Autodesk Fusion 360 part; units mm, degrees
sketch "Box" plane through (0, 0, 0) normal (0, 0, 1) x (1, 0, 0)
  line L0 (55, 25) -> (-55, 25)
  line L1 (-55, 25) -> (-55, -25)
  line L2 (-55, -25) -> (55, -25)
  line L3 (55, -25) -> (55, 25)
  line L4 (55, 25) -> (-55, -25) construction
  line L5 (-55, 25) -> (55, -25) construction
  line L6 (56, -26) -> (-56, -26)
  line L7 (-56, -26) -> (-56, 26)
  line L8 (-56, 26) -> (56, 26)
  line L9 (56, 26) -> (56, -26)
  line L10 (56, -26) -> (-56, 26) construction
  line L11 (-56, -26) -> (56, 26) construction
  dimension "d2" = 110
  dimension "d3" = 50
  dimension "d4" = 112
  dimension "d5" = 52
extrude "Extrude1" add sketch "Box" along normal blind 55
fillet "Fillet1" radius 1 4 edges at (56, -26, 27.5) (-56, -26, 27.5) (56, 26, 27.5) (-56, 26, 27.5)
fillet "Fillet2" radius 1 4 edges at (55, -25, 27.5) (55, 25, 27.5) (-55, 25, 27.5) (-55, -25, 27.5)
ref_plane "WorkPlane1" through (0, 0, 55) normal (0, 0, 1) x (1, 0, 0)
sketch "Lid" plane through (0, 0, 55) normal (0, 0, 1) x (1, 0, 0)
  line L0 (55, -26) -> (-55, -26)
  line L1 (-56, -25) -> (-56, 25)
  line L2 (-55, 26) -> (55, 26)
  line L3 (56, 25) -> (56, -25)
  line L4 (56, -26) -> (-56, 26) construction
  line L5 (-56, -26) -> (56, 26) construction
  arc A0 (-55, 26) -> (-56, 25) centre (-55, 25) ccw
  arc A1 (56, 25) -> (55, 26) centre (55, 25) ccw
  arc A2 (55, -26) -> (56, -25) centre (55, -25) ccw
  arc A3 (-56, -25) -> (-55, -26) centre (-55, -25) ccw
  dimension "d13" = 112
  dimension "d14" = 52
  dimension "d15" = 1
  dimension "d16" = 1
  dimension "d17" = 1
  dimension "d18" = 1
extrude "Extrude2" add sketch "Lid" along normal blind 2
fillet "Fillet3" radius 1 8 edges at (0, 26, 57) (-55.7071, 25.7071, 57) (-56, 0, 57) (-55.7071, -25.7071, 57) (0, -26, 57) (55.7071, -25.7071, 57) (56, 0, 57) (55.7071, 25.7071, 57)
sketch "230 plug" plane through (0, 0, 57) normal (0, 0, 1) x (-1, 0, 0)
  line L0 (-55, -25) -> (55, -25)
  line L1 (55, -25) -> (55, 25)
  line L2 (55, 25) -> (-55, 25)
  line L3 (-55, 25) -> (-55, -25)
  line L4 (8.143, -13.9073) -> (-33.857, -13.9073)
  line L5 (-33.857, 14.0927) -> (8.143, 14.0927)
  line L6 (8.143, 14.0927) -> (8.143, -13.9073)
  line L7 (8.143, -13.9073) -> (-33.857, 14.0927) construction
  line L8 (-33.857, -13.9073) -> (8.143, 14.0927) construction
  line L9 (-33.857, 14.0927) -> (-40.2209, 7.7287)
  line L10 (-33.857, 14.0927) -> (-12.0333, 14.0927) construction
  line L11 (-33.857, -13.9073) -> (-40.2209, -7.5434)
  line L12 (-33.857, -13.9073) -> (-12.0333, -13.9073) construction
  line L13 (-40.2209, -7.5434) -> (-40.2209, 7.7287)
  point P0 (-12.857, 0.0927)
  dimension "d32" = 28
  dimension "d33" = 42
  dimension "d34" = 135
  dimension "d35" = 9
  dimension "d36" = 135
  dimension "d37" = 9
extrude "Extrude3" cut sketch "230 plug" against normal blind 2 contours L4 L5 L6 L9 L11 L13
ref_plane "WorkPlane2" through (0, 0, 55) normal (0, 0, -1) x (-1, 0, 0)
sketch "Screw Holes" plane through (0, 0, 55) normal (0, 0, -1) x (1, 0, 0)
  line L0 (-8.143, 14.0927) -> (-8.143, -13.9073)
  circle A0 centre (13.857, -19.9073) radius 1.5
  line L1 (-8.143, -13.9073) -> (13.857, -13.9073)
  line L2 (13.857, -13.9073) -> (13.857, -19.9073)
  circle A1 centre (13.857, -19.9073) radius 3.5
  line L3 (-8.143, 14.0927) -> (13.857, 14.0927)
  line L4 (13.857, 14.0927) -> (13.857, 20.0927)
  circle A2 centre (13.857, 20.0927) radius 3.5
  circle A3 centre (13.857, 20.0927) radius 1.5
  dimension "d44" = 3
  dimension "d45" = 22
  dimension "d46" = 6
  dimension "d47" = 7
  dimension "d49" = 22
  dimension "d50" = 6
  dimension "d51" = 7
  dimension "d52" = 3
extrude "Extrude5" add sketch "Screw Holes" along normal blind 20
extrude "Extrude6" cut sketch "Screw Holes" against normal blind 2 contours A0 | A3
sketch "XT60 plug 1" plane through (0, 0, 55) normal (0, 0, -1) x (1, 0, 0)
  circle A0 centre (13.857, -19.9073) radius 3.5
  line L0 (40.2209, 7.7287) -> (40.2209, -7.5434)
  line L1 (40.2209, -7.5434) -> (33.857, -13.9073)
  line L2 (33.857, -13.9073) -> (-8.143, -13.9073)
  line L3 (-8.143, -13.9073) -> (-8.143, 14.0927)
  line L4 (-8.143, 14.0927) -> (33.857, 14.0927)
  line L5 (33.857, 14.0927) -> (40.2209, 7.7287)
  arc A1 (-54, 25) -> (-55, 24) centre (-54, 24) ccw
  line L6 (-55, 24) -> (-55, -24)
  arc A2 (-55, -24) -> (-54, -25) centre (-54, -24) ccw
  line L7 (-54, -25) -> (54, -25)
  arc A3 (54, -25) -> (55, -24) centre (54, -24) ccw
  line L8 (55, -24) -> (55, 24)
  arc A4 (55, 24) -> (54, 25) centre (54, 24) ccw
  line L9 (54, 25) -> (-54, 25)
  circle A5 centre (13.857, 20.0927) radius 3.5
  line L10 (-50.4445, 8.0625) -> (-42.2445, 8.0625)
  line L11 (-42.2445, -5.4375) -> (-44.8962, -8.0891)
  line L12 (-50.4445, -5.4375) -> (-47.7929, -8.0891)
  line L13 (-47.7929, -8.0891) -> (-44.8962, -8.0891)
  line L14 (-37.9445, 8.0625) -> (-29.7445, 8.0625)
  line L15 (-29.7445, 8.0625) -> (-29.7445, -5.4375)
  line L16 (-29.7445, -5.4375) -> (-32.3962, -8.0891)
  line L17 (-37.9445, -5.4375) -> (-35.2929, -8.0891)
  line L18 (-35.2929, -8.0891) -> (-32.3962, -8.0891)
  line L19 (-17.2445, 8.0625) -> (-25.4445, 8.0625)
  line L20 (-25.4445, 8.0625) -> (-25.4445, -5.4375)
  line L21 (-25.4445, -5.4375) -> (-22.7929, -8.0891)
  line L22 (-17.2445, -5.4375) -> (-19.8962, -8.0891)
  line L23 (-22.7929, -8.0891) -> (-19.8962, -8.0891)
  line L24 (-42.2445, -5.4375) -> (-42.2445, 8.0625)
  line L25 (-37.9445, -5.4375) -> (-37.9445, 8.0625)
  line L26 (-17.2445, -5.4375) -> (-17.2445, 8.0625)
  line L27 (-50.4445, 8.0625) -> (-50.4445, -5.4375)
  line L28 (-42.2445, 1.3125) -> (-37.9445, 1.3125)
  line L29 (-29.7445, 1.3125) -> (-25.4445, 1.3125)
  dimension "d70" = 3.75
  dimension "d71" = 3.75
  dimension "d72" = 8.2
  dimension "d75" = 3.75
  dimension "d76" = 3.75
  dimension "d79" = 8.2
  dimension "d80" = 13.5
  dimension "d81" = 3.75
  dimension "d83" = 3.75
  dimension "d89" = 8.2
  dimension "d91" = 4.3
extrude "Extrude7" cut sketch "XT60 plug 1" against normal blind 2 contours L19 L20 L21 L22 L23 L26 | L14 L15 L16 L17 L18 L25 | L10 L11 L12 L13 L24 L27
sketch "Sketch7" plane through (0, 0, 55) normal (0, 0, -1) x (1, 0, 0)
  line L0 (-47.7929, -8.0891) -> (-50.4445, -5.4375)
  line L1 (-50.4445, 8.0625) -> (-42.2445, 8.0625)
  line L2 (-42.2445, 8.0625) -> (-42.2445, -5.4375)
  line L3 (-42.2445, -5.4375) -> (-44.8962, -8.0891)
  line L4 (-44.8962, -8.0891) -> (-47.7929, -8.0891)
  line L5 (-29.7445, -5.4375) -> (-32.3962, -8.0891)
  line L6 (-32.3962, -8.0891) -> (-35.2929, -8.0891)
  line L7 (-35.2929, -8.0891) -> (-37.9445, -5.4375)
  line L8 (-37.9445, -5.4375) -> (-37.9445, 8.0625)
  line L9 (-37.9445, 8.0625) -> (-29.7445, 8.0625)
  line L10 (-29.7445, 8.0625) -> (-29.7445, -5.4375)
  line L11 (-25.4445, 8.0625) -> (-17.2445, 8.0625)
  line L12 (-17.2445, 8.0625) -> (-17.2445, -5.4375)
  line L13 (-17.2445, -5.4375) -> (-19.8962, -8.0891)
  line L14 (-19.8962, -8.0891) -> (-22.7929, -8.0891)
  line L15 (-22.7929, -8.0891) -> (-25.4445, -5.4375)
  line L16 (-25.4445, -5.4375) -> (-25.4445, 8.0625)
  circle A0 centre (13.857, -19.9073) radius 3.5
  line L17 (40.2209, 7.7287) -> (40.2209, -7.5434)
  line L18 (40.2209, -7.5434) -> (33.857, -13.9073)
  line L19 (33.857, -13.9073) -> (-8.143, -13.9073)
  line L20 (-8.143, -13.9073) -> (-8.143, 14.0927)
  line L21 (-8.143, 14.0927) -> (33.857, 14.0927)
  line L22 (33.857, 14.0927) -> (40.2209, 7.7287)
  arc A1 (-54, 25) -> (-55, 24) centre (-54, 24) ccw
  line L23 (-55, 24) -> (-55, -24)
  arc A2 (-55, -24) -> (-54, -25) centre (-54, -24) ccw
  line L24 (-54, -25) -> (54, -25)
  arc A3 (54, -25) -> (55, -24) centre (54, -24) ccw
  line L25 (55, -24) -> (55, 24)
  arc A4 (55, 24) -> (54, 25) centre (54, 24) ccw
  line L26 (54, 25) -> (-54, 25)
  circle A5 centre (13.857, 20.0927) radius 3.5
  line L27 (-15.2847, -9.9279) -> (-52.5832, -9.9279)
  line L28 (-52.5832, -9.9279) -> (-52.5832, 10.117)
  line L29 (-52.5832, 10.117) -> (-15.2847, 10.117)
  line L30 (-15.2847, 10.117) -> (-15.2847, -9.9279)
  line L31 (-15.2847, -9.9279) -> (-52.5832, 10.117) construction
  line L32 (-52.5832, -9.9279) -> (-15.2847, 10.117) construction
  line L33 (-50.4445, -5.4375) -> (-50.4445, 8.0625)
  point P0 (-33.934, 0.0945)
extrude "Extrude8" add sketch "Sketch7" along normal blind 14 contours L27 L28 L29 L30
extrude "Extrude4" [suppressed]
Build history of the part. All positions in model axes, mm. A direction names the side the tool comes from. Round coordinates to 2 decimals unless told otherwise and drop trailing zeros. Write each loop counter-clockwise with the first axis right and the second up, starting at its lowest first coordinate (ties: lowest second). Pieces come first, ordered by that corner, then holes. Notation, with made-up numbers: (-20, 25.25) -> (20, 25.25) arc R8 cw to (20, 30.25) -> close; hole circle Ø4 at (-35.5, 27). An arc over 180 degrees is marked (long way). Write item = value, one per line.
(1) Band-saw the part on C-C (z = 16.5). Give the cut face in (x, y), then the cut area to 3 significant figures.
Answer:
outline = (-56, -25) arc R1 ccw to (-55, -26) -> (55, -26) arc R1 ccw to (56, -25) -> (56, 25) arc R1 ccw to (55, 26) -> (-55, 26) arc R1 ccw to (-56, 25) -> close; hole (-55, -24) arc R1 ccw to (-54, -25) -> (54, -25) arc R1 ccw to (55, -24) -> (55, 24) arc R1 ccw to (54, 25) -> (-54, 25) arc R1 ccw to (-55, 24) -> close
area = 324 mm2
(2) Tool access for faces 3 (the face through (-0.3, 25.2, 0)), 4 (the face through (-46, -8.062, 49)), 5 (the face through (-34, -10.117, 48)): list every direction of +Z, -Z, +X, -X, +Y, -Y with a clear straight run to the whole face (end or side of a thin tool).
Answer:
face_3 = -Z, +X, -X, +Y, -Y
face_4 = +Z, -Z
face_5 = -Z
(3) Two-plate mould, pull along Y, no slides. Class faces 1 (the face through (56, 0, 28)), 2 (the face through (-34, 9.928, 48)): pulls with the +Y half, pulls with the -Y half, needs draft (parallel to the pull), parting line crosses it, or undercut.
Answer:
face_1 = needs draft
face_2 = undercut
(4) Flat gauge pins, fed straight in: pin 1 (3.5 mm diameter, centred on x = 14.5, y = -21.5, fed in from -Z); pin 2 (6 mm diameter, centred on x = -40, y = 2, fed in from -Z). Where does each tip first touch, or does it go through?
Answer:
pin_1 = 35
pin_2 = 41
(5) Band-saw the part on D-D (z = 38.5). Give the cut face in (x, y), then the cut area to 3 significant figures.
Answer:
outline = (-56, -25) arc R1 ccw to (-55, -26) -> (55, -26) arc R1 ccw to (56, -25) -> (56, 25) arc R1 ccw to (55, 26) -> (-55, 26) arc R1 ccw to (-56, 25) -> close; circle Ø7 at (13.86, -20.09); circle Ø7 at (13.86, 19.91); hole (-55, -24) arc R1 ccw to (-54, -25) -> (54, -25) arc R1 ccw to (55, -24) -> (55, 24) arc R1 ccw to (54, 25) -> (-54, 25) arc R1 ccw to (-55, 24) -> close; hole circle Ø3 at (13.86, -20.09); hole circle Ø3 at (13.86, 19.91)
area = 387 mm2
(6) Band-saw the part on A-A (y = 2). State how many separate pieces and enclosed holes the cut face has, then the cut area to 3 significant figures.
Answer:
separate_pieces = 5
enclosed_holes = 0
area = 365 mm2
(7) Probe L1, parallel to Y at x = -40, z = 50; L2, parallel to X at y = -16, z = 7; L3, parallel to Y at x = 30.5, z = 42. List the from-to ranges inside material, lowest first.
Answer:
L1 = -26 to -25, -10.12 to 9.93, 25 to 26
L2 = -56 to -55, 55 to 56
L3 = -26 to -25, 25 to 26
(8) Band-saw the part on B-B (x = 27). Give the cut face in (y, z).
Answer:
outline = (-26, 0) -> (-25, 0) -> (-25, 55) -> (-14.09, 55) -> (-14.09, 57) -> (-25, 57) arc R1 ccw to (-26, 56) -> close; (13.91, 55) -> (25, 55) -> (25, 0) -> (26, 0) -> (26, 56) arc R1 ccw to (25, 57) -> (13.91, 57) -> close
